Design review of the part built by this model. Coordinates are the model's own, in mm. Give positions to 0.01 mm unless a question says otherwise; leave off trailing zeros. Write each loop counter-clockwise with the first axis right and the second up, starting at its lowest first coordinate (ties: lowest second). Pieces come first, ordered by that corner, then holes. Notation, with made-up numbers: M 1.25,76.5 L 24.25,76.5 A15 cw 24.25,97.5 Z; hole C -1.5,12.5 d9. An arc over 180 degrees is marked long. Answer in a Markdown table with one row per item.
```python
from build123d import *

# Parameters (mm, degrees)
F0_W     = 200
F0_H     = 1500
F0_W_2   = 100
F0_H_2   = 28
F1_DEPTH = 10
F2_W     = 200
F2_H     = 1500
F2_W_2   = 100
F2_H_2   = 28
F3_DEPTH = 6
F5_DEPTH = 68
F6_W     = 168
F6_H     = 1380
F7_DEPTH = 16
F8_R     = 2


# Not quite as in the source:
# - a feature names something its author has since deleted; it is built from what else it names


with BuildPart() as f1:
    # F0 (on Front) → F1 (new body)
    with BuildSketch(Plane.XZ):
        with Locations((0, -2.5)):
            Rectangle(F0_W, F0_H)
        with Locations((0, -93.5)):
            Rectangle(F0_W_2, F0_H_2, mode=Mode.SUBTRACT)
        with Locations((0, -48.5)):
            Rectangle(F0_W_2, F0_H_2, mode=Mode.SUBTRACT)
        with Locations((0, -3.5)):
            Rectangle(F0_W_2, F0_H_2, mode=Mode.SUBTRACT)
        with Locations((0, 41.5)):
            Rectangle(F0_W_2, F0_H_2, mode=Mode.SUBTRACT)
        with Locations((0, 86.5)):
            Rectangle(F0_W_2, F0_H_2, mode=Mode.SUBTRACT)
        with Locations((0, 131.5)):
            Rectangle(F0_W_2, F0_H_2, mode=Mode.SUBTRACT)
        with Locations((0, 176.5)):
            Rectangle(F0_W_2, F0_H_2, mode=Mode.SUBTRACT)
        with Locations((0, 221.5)):
            Rectangle(F0_W_2, F0_H_2, mode=Mode.SUBTRACT)
        with Locations((0, 266.5)):
            Rectangle(F0_W_2, F0_H_2, mode=Mode.SUBTRACT)
        with Locations((0, 311.5)):
            Rectangle(F0_W_2, F0_H_2, mode=Mode.SUBTRACT)
        with Locations((0, 356.5)):
            Rectangle(F0_W_2, F0_H_2, mode=Mode.SUBTRACT)
        with Locations((0, 401.5)):
            Rectangle(F0_W_2, F0_H_2, mode=Mode.SUBTRACT)
        with Locations((0, 446.5)):
            Rectangle(F0_W_2, F0_H_2, mode=Mode.SUBTRACT)
        with Locations((0, 491.5)):
            Rectangle(F0_W_2, F0_H_2, mode=Mode.SUBTRACT)
        with Locations((0, 536.5)):
            Rectangle(F0_W_2, F0_H_2, mode=Mode.SUBTRACT)
    extrude(amount=F1_DEPTH)

    # F2 (on face) → F3 (join)
    with BuildSketch(Plane(origin=(0, 0, 0), x_dir=(-1, 0, 0), z_dir=(0, 1, 0))):
        with Locations((0, -2.5)):
            Rectangle(F2_W, F2_H)
        with Locations((0, -93.5)):
            Rectangle(F2_W_2, F2_H_2, mode=Mode.SUBTRACT)
        with Locations((0, -48.5)):
            Rectangle(F2_W_2, F2_H_2, mode=Mode.SUBTRACT)
        with Locations((0, -3.5)):
            Rectangle(F2_W_2, F2_H_2, mode=Mode.SUBTRACT)
        with Locations((0, 41.5)):
            Rectangle(F2_W_2, F2_H_2, mode=Mode.SUBTRACT)
        with Locations((0, 86.5)):
            Rectangle(F2_W_2, F2_H_2, mode=Mode.SUBTRACT)
        with Locations((0, 131.5)):
            Rectangle(F2_W_2, F2_H_2, mode=Mode.SUBTRACT)
        with Locations((0, 176.5)):
            Rectangle(F2_W_2, F2_H_2, mode=Mode.SUBTRACT)
        with Locations((0, 221.5)):
            Rectangle(F2_W_2, F2_H_2, mode=Mode.SUBTRACT)
        with Locations((0, 266.5)):
            Rectangle(F2_W_2, F2_H_2, mode=Mode.SUBTRACT)
        with Locations((0, 311.5)):
            Rectangle(F2_W_2, F2_H_2, mode=Mode.SUBTRACT)
        with Locations((0, 356.5)):
            Rectangle(F2_W_2, F2_H_2, mode=Mode.SUBTRACT)
        with Locations((0, 401.5)):
            Rectangle(F2_W_2, F2_H_2, mode=Mode.SUBTRACT)
        with Locations((0, 446.5)):
            Rectangle(F2_W_2, F2_H_2, mode=Mode.SUBTRACT)
        with Locations((0, 491.5)):
            Rectangle(F2_W_2, F2_H_2, mode=Mode.SUBTRACT)
        with Locations((0, 536.5)):
            Rectangle(F2_W_2, F2_H_2, mode=Mode.SUBTRACT)
        with Locations((0, -93.5)):
            Rectangle(F2_W_2, F2_H_2)
        with Locations((0, -48.5)):
            Rectangle(F2_W_2, F2_H_2)
        with Locations((0, -3.5)):
            Rectangle(F2_W_2, F2_H_2)
        with Locations((0, 41.5)):
            Rectangle(F2_W_2, F2_H_2)
        with Locations((0, 86.5)):
            Rectangle(F2_W_2, F2_H_2)
        with Locations((0, 131.5)):
            Rectangle(F2_W_2, F2_H_2)
        with Locations((0, 176.5)):
            Rectangle(F2_W_2, F2_H_2)
        with Locations((0, 221.5)):
            Rectangle(F2_W_2, F2_H_2)
        with Locations((0, 266.5)):
            Rectangle(F2_W_2, F2_H_2)
        with Locations((0, 311.5)):
            Rectangle(F2_W_2, F2_H_2)
        with Locations((0, 356.5)):
            Rectangle(F2_W_2, F2_H_2)
        with Locations((0, 401.5)):
            Rectangle(F2_W_2, F2_H_2)
        with Locations((0, 446.5)):
            Rectangle(F2_W_2, F2_H_2)
        with Locations((0, 491.5)):
            Rectangle(F2_W_2, F2_H_2)
        with Locations((0, 536.5)):
            Rectangle(F2_W_2, F2_H_2)
    extrude(amount=F3_DEPTH)

    # F4 (on face) → F5 (join)
    with BuildSketch(Plane(origin=(0, 6, 0), x_dir=(-1, 0, 0), z_dir=(0, 1, 0))):
        Polygon((100, 747.5), (-100, 747.5), (-100, 627.5), (-100, -752.5), (-84, -752.5), (-84, -732.5), (-84, 627.5), (84, 627.5), (84, -732.5), (84, -752.5), (100, -752.5), (100, 727.5), align=None)
    extrude(amount=F5_DEPTH)

    # F6 (on face) → F7 (join)
    with BuildSketch(Plane(origin=(0, 74, 0), x_dir=(-1, 0, 0), z_dir=(0, 1, 0))):
        Polygon((100, 747.5), (-100, 747.5), (-100, -752.5), (-84, -752.5), (-84, 627.5), (84, 627.5), (84, -752.5), (100, -752.5), align=None)
        with Locations((0, -62.5)):
            Rectangle(F6_W, F6_H)
    extrude(amount=F7_DEPTH)

    # F8
    f8_edges = [f1.edges().sort_by_distance(p)[0] for p in [
        (100, 40, -752.5),
        (100, -10, -2.5),
        (100, 40, 747.5),
        (100, 90, -2.5),
        (-100, -10, -2.5),
        (-100, 40, -752.5),
        (-100, 90, -2.5),
        (-100, 40, 747.5),
        (0, -10, 747.5),
        (0, -10, -752.5),
        (0, -10, -107.5),
        (-50, -10, -93.5),
        (0, -10, -79.5),
        (50, -10, -93.5),
        (0, -10, -62.5),
        (-50, -10, -48.5),
        (0, -10, -34.5),
        (50, -10, -48.5),
        (0, -10, -17.5),
        (-50, -10, -3.5),
        (0, -10, 10.5),
        (50, -10, -3.5),
        (0, -10, 27.5),
        (-50, -10, 41.5),
        (0, -10, 55.5),
        (50, -10, 41.5),
        (0, -10, 72.5),
        (-50, -10, 86.5),
        (0, -10, 100.5),
        (50, -10, 86.5),
        (0, -10, 117.5),
        (-50, -10, 131.5),
        (0, -10, 145.5),
        (50, -10, 131.5),
        (0, -10, 162.5),
        (-50, -10, 176.5),
        (0, -10, 190.5),
        (50, -10, 176.5),
        (0, -10, 207.5),
        (-50, -10, 221.5),
        (0, -10, 235.5),
        (50, -10, 221.5),
        (0, -10, 252.5),
        (-50, -10, 266.5),
        (0, -10, 280.5),
        (50, -10, 266.5),
        (0, -10, 297.5),
        (-50, -10, 311.5),
        (0, -10, 325.5),
        (50, -10, 311.5),
        (0, -10, 342.5),
        (-50, -10, 356.5),
        (0, -10, 370.5),
        (50, -10, 356.5),
        (0, -10, 387.5),
        (-50, -10, 401.5),
        (0, -10, 415.5),
        (50, -10, 401.5),
        (0, -10, 432.5),
        (-50, -10, 446.5),
        (0, -10, 460.5),
        (50, -10, 446.5),
        (0, -10, 477.5),
        (-50, -10, 491.5),
        (0, -10, 505.5),
        (50, -10, 491.5),
        (0, -10, 522.5),
        (-50, -10, 536.5),
        (0, -10, 550.5),
        (50, -10, 536.5),
        (0, 90, 747.5),
        (0, 90, -752.5),
    ]]
    fillet(f8_edges, radius=F8_R)


solid = f1.part
```
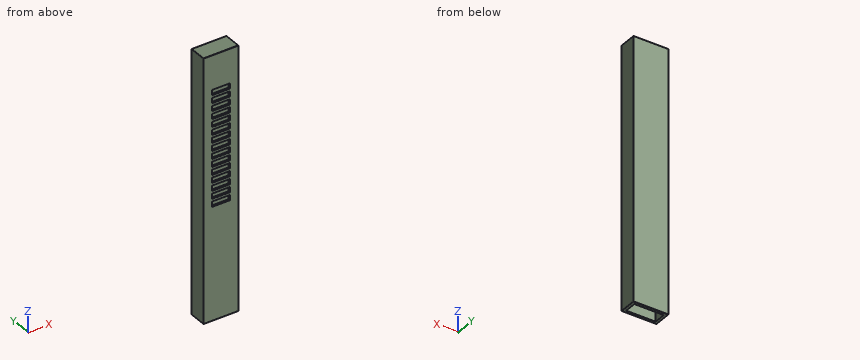
1) Insertion check: P1, Ø14, axis at x = -21.5, z = -88.5, coming from the -Y side; P2, Ø8, axis at x = 8.5, z = 143, coming from the -Y side. Each pin has a flat end and moves straight along its axis. Give the tip position at first contact, or say it passes through.
Geometry says:
| item | result |
|---|---|
| P1 | y = 0 |
| P2 | y = -9.94 |
2) Add section A-A (z = -649.5). Write out the cut boundary in (x, y).
Geometry says:
| item | result |
|---|---|
| outline | M -100,-8 A2 ccw -98,-10 L 98,-10 A2 ccw 100,-8 L 100,88 A2 ccw 98,90 L -98,90 A2 ccw -100,88 Z; hole M -84,6 L 84,6 L 84,74 L -84,74 Z |
3) Add section C-C (x = 66.5). Write out the cut boundary in (y, z).
Geometry says:
| item | result |
|---|---|
| outline | M -10,-750.5 A2 ccw -8,-752.5 L 6,-752.5 L 6,627.5 L 74,627.5 L 74,-752.5 L 88,-752.5 A2 ccw 90,-750.5 L 90,745.5 A2 ccw 88,747.5 L -8,747.5 A2 ccw -10,745.5 Z |
4) Add section B-B (y = 60.5). Write out the cut boundary in (x, z).
Geometry says:
| item | result |
|---|---|
| outline | M -100,-750.5 A2 ccw -98,-752.5 L -84,-752.5 L -84,627.5 L 84,627.5 L 84,-752.5 L 98,-752.5 A2 ccw 100,-750.5 L 100,745.5 A2 ccw 98,747.5 L -98,747.5 A2 ccw -100,745.5 Z |
5) To check wall thickness, follow probe 1 along X at (y, z) = (46, -7.5); probe 2 along Y at (x, z) = (55, 493); probe 3 along Z at (x, y) = (80.5, 50). State the ranges of each line that lie inside material, in increasing order. Write a range as [from, to].
Geometry says:
| item | result |
|---|---|
| probe 1 | [-100, -84], [84, 100] |
| probe 2 | [-10, 6], [74, 90] |
| probe 3 | [627.5, 747.5] |
